Could you check a few things on this drawing? It's one solid part, dimensions in mm from its lowest x, y, z. A direction names the side the tool comes from. Give positions to 0.01 mm unless a question says otherwise; leave off trailing zeros. Order: outer loops, then holes, each group sorted by start corner. A loop starts at its lowest first (then second) coordinate and runs counter-clockwise, first axis right, second up. Notation, with made-up numbers: (73, 11.25) -> (112, 11.25) arc R31 cw to (112, 48.25) -> close; hole circle Ø1 at (71, 6.5). An arc over 180 degrees is marked (long way). Write each question's results on one line, items separated by ' | '. Start each with the question number.
Q1. I'm going to push flat-ended pins straight in: pin 1 (1 mm diameter, centred on x = 28, z = 1.5, fed in from -Y); pin 2 (6 mm diameter, centred on x = 11, y = 22, fed in from -Z). Where does each tip first touch, or does it pass through?
Q2. Imagine slicing it at C-C, the plane z = 3.25. Please give me the cut outline in (x, y), then the cut area to 3 significant figures.
Q3. Thinking about a two-plate mould opening in Y: for the marked faces 1, 2 and 3, which applies, pulls with the +Y half, pulls with the -Y half, needs draft (parallel to the pull), parting line crosses it, or undercut?
Q4. Imagine slicing it at A-A, the plane x = 34.2. Please give me the cut outline in (y, z).
Q5. I need wall thicknesses on line 1 along X through (y, z) = (20.75, 1); line 2 along Y through (x, z) = (3, 0.75); line 3 along Z through (x, y) = (34, 12). Which ranges of each line are inside material? Lowest first, please. Write a range as [from, to].
Q6. Imagine slicing it at B-B, the plane y = 4.6. Please give me the cut outline in (x, z).
Q7. For the marked faces 4 and 5, which set-ups out of +Z, -Z, +X, -X, +Y, -Y let a thin tool reach every point of the face, with its end or its side?
Q8. Imagine slicing it at D-D, the plane y = 25. Please give me the cut outline in (x, z).
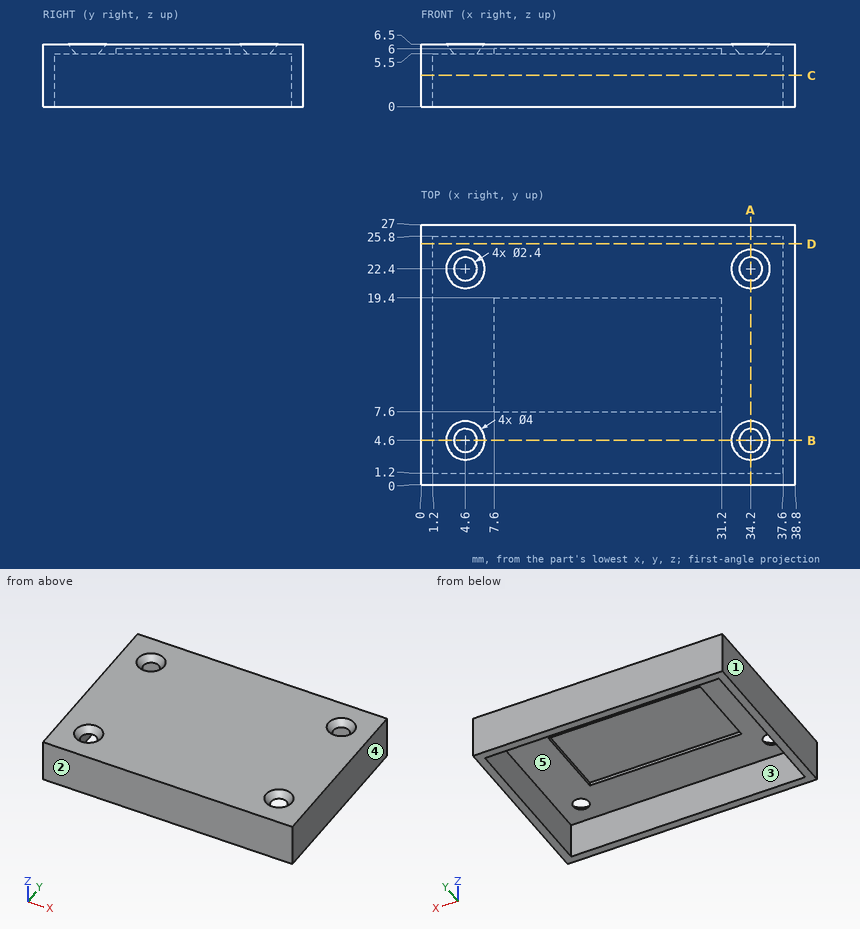
Geometry check:
1) pin 1: y = 0 | pin 2: z = 5.5
2) outline: (0, 0) -> (38.8, 0) -> (38.8, 27) -> (0, 27) -> close; hole (1.2, 1.2) -> (37.6, 1.2) -> (37.6, 25.8) -> (1.2, 25.8) -> close | area: 152 mm²
3) face 1: needs draft | face 2: pulls with the -Y half | face 3: undercut
4) outline: (0, 0) -> (1.2, 0) -> (1.2, 5.5) -> (3.4, 5.5) -> (2.6, 6.5) -> (0, 6.5) -> close; (5.8, 5.5) -> (21.2, 5.5) -> (20.4, 6.5) -> (6.6, 6.5) -> close; (23.6, 5.5) -> (25.8, 5.5) -> (25.8, 0) -> (27, 0) -> (27, 6.5) -> (24.4, 6.5) -> close
5) line 1: [0, 1.2], [37.6, 38.8] | line 2: [0, 1.2], [25.8, 27] | line 3: [5.5, 6.5]
6) outline: (0, 0) -> (1.2, 0) -> (1.2, 5.5) -> (3.4, 5.5) -> (2.6, 6.5) -> (0, 6.5) -> close; (5.8, 5.5) -> (33, 5.5) -> (32.2, 6.5) -> (6.6, 6.5) -> close; (35.4, 5.5) -> (37.6, 5.5) -> (37.6, 0) -> (38.8, 0) -> (38.8, 6.5) -> (36.2, 6.5) -> close
7) face 4: +Z, -Z, +X, +Y, -Y | face 5: -Z
8) outline: (0, 0) -> (1.2, 0) -> (1.2, 5.5) -> (37.6, 5.5) -> (37.6, 0) -> (38.8, 0) -> (38.8, 6.5) -> (0, 6.5) -> close
